Study the drawing (mm; zero at the part's minimum x, y, z) and answer. Coordinates: 2 decimals unless noted, no trailing zeros. Order: outer loops, then holes, each group sorted by start corner. A loop starts at its lowest first (then second) coordinate and runs counter-clockwise, first axis right, second up. Notation, with made-up numbers: (71.5, 52.25) -> (107.5, 52.25) arc R21 cw to (107.5, 81.25) -> close; hole circle Ø5 at (51, 73). An arc over 180 degrees is marked (long way). Answer in a Markdown table with one row per item. Add a question column.
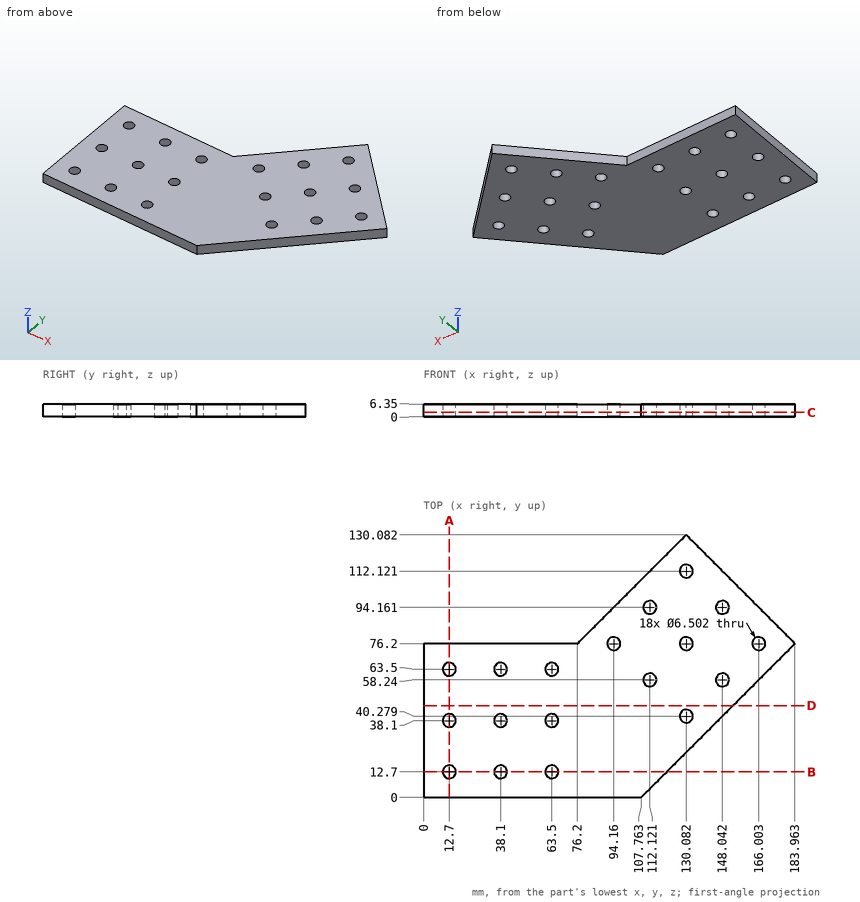
Q1. A cutting plane is placed at A-A (x = 12.7). Determine the outline of the cut face in (y, z).
Q2. Straight lines are drawn through the part: line 1 (Y direction, x = 63.5, z = 3); line 2 (Y direction, x = 12.5, z = 3.25) (1 decimal); line 3 (Y direction, x = 150, z = 4) (1 decimal). For each, find the intervals that lie inside material, in ascending order.
Q3. A cutting plane is placed at D-D (y = 45.5). Determine the outline of the cut face in (x, z).
Q4. Given pin 1 (3 mm diameter, centred on x = 34, z = 4, fed in from +Y); pin 2 (3 mm diameter, centred on y = 70.5, z = 1.5, fed in from +X) (1 decimal), each flat-ended and moving along its own axis, determine where each tip first touches the part or whether it passes through.
Q5. A cutting plane is placed at C-C (z = 2.25). State how many separate pieces and enclosed holes the cut face has, then the cut area to 3 significant figures.
Q6. A cutting plane is placed at B-B (y = 12.7). Determine the outline of the cut face in (x, z).
Returned:
| question | item | result |
|---|---|---|
| 1 | outline | (0, 0) -> (9.45, 0) -> (9.45, 6.35) -> (0, 6.35) -> close; (15.95, 0) -> (34.85, 0) -> (34.85, 6.35) -> (15.95, 6.35) -> close; (41.35, 0) -> (60.25, 0) -> (60.25, 6.35) -> (41.35, 6.35) -> close; (66.75, 0) -> (76.2, 0) -> (76.2, 6.35) -> (66.75, 6.35) -> close |
| 2 | line 1 | y = 0 to 9.45, 15.95 to 34.85, 41.35 to 60.25, 66.75 to 76.2 |
| 2 | line 2 | y = 0 to 9.5, 15.9 to 34.9, 41.3 to 60.3, 66.7 to 76.2 |
| 2 | line 3 | y = 42.2 to 55.6, 60.8 to 91.6, 96.8 to 110.2 |
| 3 | outline | (0, 0) -> (153.26, 0) -> (153.26, 6.35) -> (0, 6.35) -> close |
| 4 | pin 1 | stops at y = 76.2 |
| 4 | pin 2 | stops at x = 179.8 |
| 5 | separate pieces | 1 |
| 5 | enclosed holes | 18 |
| 5 | area | 13,400 mm² |
| 6 | outline | (0, 0) -> (9.45, 0) -> (9.45, 6.35) -> (0, 6.35) -> close; (15.95, 0) -> (34.85, 0) -> (34.85, 6.35) -> (15.95, 6.35) -> close; (41.35, 0) -> (60.25, 0) -> (60.25, 6.35) -> (41.35, 6.35) -> close; (66.75, 0) -> (120.46, 0) -> (120.46, 6.35) -> (66.75, 6.35) -> close |
